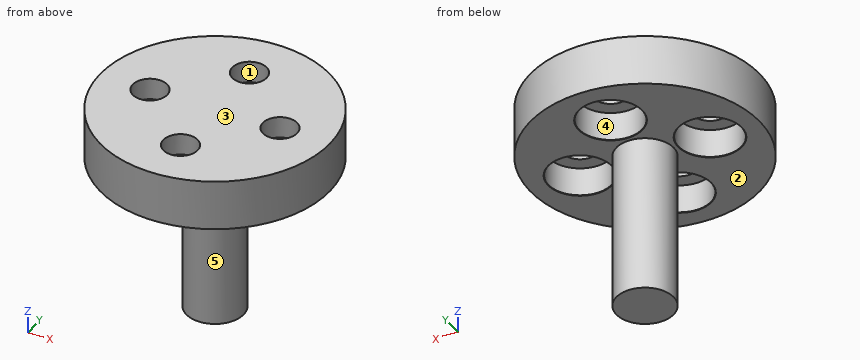
from build123d import *

# Parameters (mm, degrees)
CBORE_FOR_M2_SHCS1_AT_2_COUNT = 2
CBORE_FOR_M2_SHCS1_AT_2_PITCH = 6.363961031
CBORE_FOR_M2_SHCS1_AT_3_COUNT = 2
CBORE_FOR_M2_SHCS1_AT_3_PITCH = 9
CBORE_FOR_M2_SHCS1_AT_4_COUNT = 2
CBORE_FOR_M2_SHCS1_AT_4_PITCH = 6.363961031


with BuildPart() as part:
    # Sketch2 → Revolve1 (revolve)
    with BuildSketch(Plane(origin=(0, 0, 0), x_dir=(1, 0, 0), z_dir=(0, 1, 0)), mode=Mode.PRIVATE) as revolve1_sk:
        Polygon((0, 0), (8, 0), (8, 3.5), (2, 3.5), (2, 14.5), (0, 14.5), align=None)
    revolve(revolve1_sk.sketch.rotate(Axis((0, 0, -14.5), (0, 0, 1)), 180), axis=Axis((0, 0, -14.5), (0, 0, 1)))

    # Sketch5 → CBORE for M2 SHCS1 (revolve, cut)
    with BuildSketch(Plane(origin=(0, 4.5, -3.5), x_dir=(0, 1, 0), z_dir=(1, 0, 0))):
        Polygon((0, 0), (0, 3.5), (1.2, 3.5), (1.2, 2), (2.2, 2), (2.2, 0.020977491), (2.225, 0), align=None)
    cbore_for_m2_shcs1 = revolve(axis=Axis((0, 4.5, -9.85), (0, 0, 1)), mode=Mode.SUBTRACT)

    # CBORE for M2 SHCS1 at 2: CBORE for M2 SHCS1 ×2
    with Locations(*[Vector(-0.7071067811865476, -0.7071067811865476, 0) * (i * CBORE_FOR_M2_SHCS1_AT_2_PITCH) for i in range(1, CBORE_FOR_M2_SHCS1_AT_2_COUNT)]):
        add(cbore_for_m2_shcs1, mode=Mode.SUBTRACT)

    # CBORE for M2 SHCS1 at 3: CBORE for M2 SHCS1 ×2
    with Locations(*[(0, -i * CBORE_FOR_M2_SHCS1_AT_3_PITCH, 0) for i in range(1, CBORE_FOR_M2_SHCS1_AT_3_COUNT)]):
        add(cbore_for_m2_shcs1, mode=Mode.SUBTRACT)

    # CBORE for M2 SHCS1 at 4: CBORE for M2 SHCS1 ×2
    with Locations(*[Vector(0.7071067811865476, -0.7071067811865476, 0) * (i * CBORE_FOR_M2_SHCS1_AT_4_PITCH) for i in range(1, CBORE_FOR_M2_SHCS1_AT_4_COUNT)]):
        add(cbore_for_m2_shcs1, mode=Mode.SUBTRACT)


solid = part.part
Input: part model. Units: mm. Frame: model coordinates. Face numbers are marked on the shaded views. A direction names the side the tool comes from. Give positions to 0.01 mm unless a question says otherwise; leave off trailing zeros. Write each loop counter-clockwise with the first axis right and the second up, starting at its lowest first coordinate (ties: lowest second). Pieces come first, ordered by that corner, then holes. Notation, with made-up numbers: M -5,-35.5 L 34,-35.5 A27 ccw 34,-6.5 Z; hole C -40,-0.75 d2. An arc over 180 degrees is marked long. Use one line per item in the form item = value.
1. First-contact query: P1, Ø4, axis at x = -4.5, y = 0, coming from the -Z side; P2, Ø3.5, axis at x = -5, y = 1, coming from the -Z side; P3, Ø5, axis at x = 4, y = 0.5, coming from the -Z side; P4, Ø4, axis at y = 5, z = -5, coming from the +X side. Flat tips, straight axial feed; report the tip coordinate or a pass-through.
Outcome:
P1 = -1.5
P2 = -3.5
P3 = -14.5
P4 = 7.1
2. Cut plane B-B on z = -1.25. Return loops of the section in (x, y), and give its area (3 significant figures).
Outcome:
outline = C 0,0 d16; hole C -4.5,0 d2.4; hole C 0,-4.5 d2.4; hole C 0,4.5 d2.4; hole C 4.5,0 d2.4
area = 183 mm²
3. Cut plane A-A on y = 0. Return loops of the section in (x, z) (3 decimals), and give its area (3 significant figures).
Outcome:
outline = M -8,-3.5 L -6.725,-3.5 L -6.7,-3.479 L -6.7,-1.5 L -5.7,-1.5 L -5.7,0 L -8,0 Z; M -3.3,-1.5 L -2.3,-1.5 L -2.3,-3.479 L -2.275,-3.5 L -2,-3.5 L -2,-14.5 L 2,-14.5 L 2,-3.5 L 2.275,-3.5 L 2.3,-3.479 L 2.3,-1.5 L 3.3,-1.5 L 3.3,0 L -3.3,0 Z; M 5.7,-1.5 L 6.7,-1.5 L 6.7,-3.479 L 6.725,-3.5 L 8,-3.5 L 8,0 L 5.7,0 Z
area = 75.2 mm²
4. Mould query, pull axis X, two halves, no side actions, for the marked faces 3, 4 and 5. Classes: released by +X, released by -X, zero draft, split by the parting line, or undercut.
Outcome:
face_3 = zero draft
face_4 = undercut
face_5 = split by the parting line
5. Ray query, L1, parallel to Y at x = 0, z = -2.15; L2, parallel to Y at x = 0, z = -0.95; L3, parallel to Z at x = 1.5, y = -4.5. Return the intervals inside material, ascending.
Outcome:
L1 = -8 to -6.7, -2.3 to 2.3, 6.7 to 8
L2 = -8 to -5.7, -3.3 to 3.3, 5.7 to 8
L3 = -1.5 to 0
6. Cut plane C-C on x = -4.5. Return loops of the section in (y, z) (3 decimals), and give its area (3 significant figures).
Outcome:
outline = M -6.614,-3.5 L -2.225,-3.5 L -2.2,-3.479 L -2.2,-1.5 L -1.2,-1.5 L -1.2,0 L -6.614,0 Z; M 1.2,-1.5 L 2.2,-1.5 L 2.2,-3.479 L 2.225,-3.5 L 6.614,-3.5 L 6.614,0 L 1.2,0 Z
area = 33.9 mm²
7. Reachability of the marked faces 1 and 2 from +Z, -Z, +X, -X, +Y, -Y: full face, straight path, thin tool, end or side. Return the list, or none.
Outcome:
face_1 = +Z, -Z
face_2 = -Z
